Input: part model. Units: mm. Frame: model coordinates. A direction names the side the tool comes from. Coordinates: 2 decimals unless noted, no trailing zeros. Write each loop counter-clockwise with the first axis right and the second up, starting at its lowest first coordinate (ties: lowest second). Pieces come first, ordered by that corner, then holes. Notation, with made-up numbers: M 45.25,-1 L 86.25,-1 A10 ccw 86.25,3 Z; hole C 68.25,9 d5. An arc over 180 degrees is marked long. Use CSV: the item, a comma, the result in double quotes.
Autodesk Inventor part; units mm, degrees
ref_plane "YZ Plane" through (0, 0, 0) normal (1, 0, 0) x (0, 1, 0)
ref_plane "XZ Plane" through (0, 0, 0) normal (0, 1, 0) x (-1, 0, 0)
ref_plane "XY Plane" through (0, 0, 0) normal (0, 0, 1) x (1, 0, 0)
sketch "esq_rev" plane through (0, 0, 0) normal (0, 0, 1) x (1, 0, 0)
  line L0 (0, -38.1) -> (0, 50.1)
  line L1 (7.5, -9.5) -> (7.5, 9.5)
  line L2 (7.5, 9.5) -> (13, 9.5)
  line L3 (13, 9.5) -> (13, 22.5)
  line L4 (13, 22.5) -> (30, 22.5)
  line L5 (30, 22.5) -> (30, 37.5)
  line L6 (30, 37.5) -> (0, 37.5)
  line L7 (0, -25.5) -> (0, -0.0006)
  line L8 (-38.091, 0) -> (41.3485, 0)
  line L9 (-26.7425, 30) -> (-5.3911, 30)
  line L10 (-5.3911, 30) -> (28.4337, 30)
  line L11 (28.4337, 30) -> (7.0823, 30)
  line L12 (7.0823, 30) -> (-26.7425, 30)
  line L13 (-6.854, 30) -> (-23.5883, 30)
  line L14 (-23.5883, 30) -> (-14.3845, 30)
  line L15 (-4.5388, 30) -> (-6.854, 30)
  line L16 (-24.4454, 30) -> (5.2291, 30)
  line L17 (5.2291, 30) -> (2.6006, 30)
  line L18 (-13.9964, 30) -> (-24.4454, 30)
  line L19 (24.4454, 30) -> (-5.2291, 30)
  line L20 (-5.2291, 30) -> (-2.6006, 30)
  line L21 (13.9964, 30) -> (24.4454, 30)
  line L22 (4.5388, 30) -> (7.194, 30)
  line L23 (7.194, 30) -> (24.9396, 30)
  line L24 (24.9396, 30) -> (14.3845, 30)
  line L25 (-4.5388, 30) -> (-14.5, 30)
  line L26 (2.6006, 30) -> (-13.9964, 30)
  line L27 (13.9964, 30) -> (-2.6006, 30)
  line L28 (14.5, 30) -> (4.5388, 30)
  line L29 (-12.5, 30) -> (12.5, 30)
  line L30 (-12.5, -20) -> (12.5, -20)
  line L31 (7, -9.5) -> (7, -25.5)
  line L32 (7, -25.5) -> (0, -25.5)
  line L33 (7, -9.5) -> (7.5, -9.5)
  line L34 (0, -0.0006) -> (0, 37.5)
  point P0 (0, 0)
  dimension "d0" = 30
  dimension "d1" = 13
  dimension "d2" = 7.5
  dimension "d5" = 13
  dimension "d6" = 15
  dimension "d23" = 7
  dimension "d25" = 19
  dimension "d26" = 16
revolve "rev" add sketch "esq_rev" angle 360 about axis through (0, -25.5, 0) along (0, 1, 0)
sketch "esq_percage" plane through (0, 0, 0) normal (0, 1, 0) x (-1, 0, 0)
  line L0 (0, -7) -> (0, 7)
  line L1 (-7, 0) -> (7, 0)
  circle A0 centre (0, 0) radius 5
  dimension "d8" = 10
extrude "ext_percage" cut sketch "esq_percage" along normal through all both and the other way through all
sketch "Esq_trous" plane through (0, 0, 0) normal (0, 1, 0) x (-1, 0, 0)
  line L0 (0, -4.9) -> (0, 29.4)
  line L1 (-3.5, 0) -> (3.5, 0)
  circle A0 centre (0, 22) radius 2.5
  point P0 (0, 0)
  dimension "d11" = 5
  dimension "d12" = 22
extrude "ext_trous" cut sketch "Esq_trous" along normal through all
pattern_circular "Réseau circulaire1" count 6 over 360 about axis through (0, -10, 0) along (0, 1, 0) of "ext_trous"
thread "Filetage2"
properties part number "wheel_hub_spacer" material "Aluminium 6061"
1. Section A-A (z = 0). Return loops of the section in (x, y), then the cut area to 3 significant figures.
Resolved:
outline,"M -30,22.5 L -13,22.5 L -13,9.5 L -7.5,9.5 L -7.5,-9.5 L -7,-9.5 L -7,-25.5 L -5,-25.5 L -5,37.5 L -30,37.5 Z; M 5,-25.5 L 7,-25.5 L 7,-9.5 L 7.5,-9.5 L 7.5,9.5 L 13,9.5 L 13,22.5 L 30,22.5 L 30,37.5 L 5,37.5 Z"
area,"1,120 mm^2"
2. Section B-B (x = 0). Return loops of the section in (y, z), then the cut area to 3 significant figures.
Resolved:
outline,"M -25.5,-7 L -9.5,-7 L -9.5,-7.5 L 9.5,-7.5 L 9.5,-13 L 22.5,-13 L 22.5,-19.5 L 37.5,-19.5 L 37.5,-5 L -25.5,-5 Z; M -25.5,5 L 37.5,5 L 37.5,19.5 L 22.5,19.5 L 22.5,13 L 9.5,13 L 9.5,7.5 L -9.5,7.5 L -9.5,7 L -25.5,7 Z; M 22.5,-30 L 37.5,-30 L 37.5,-24.5 L 22.5,-24.5 Z; M 22.5,24.5 L 37.5,24.5 L 37.5,30 L 22.5,30 Z"
area,"967 mm^2"
3. Mould query, pull axis X, two halves, no side actions, for faces 1 (the flat face through (-2, -25.5, -5)), 2 (the cylindrical face through (-19.59, 29.9, 8.56)), 3 (the cylindrical face through (6.466, -17.612, -2.681)). Classes: pulls with the +X half, pulls with the -X half, needs draft (parallel to the pull), parting line crosses it, or undercut.
Resolved:
face 1,"needs draft"
face 2,"undercut"
face 3,"parting line crosses it"
4. Section D-D (y = 30). Return loops of the section in (x, z).
Resolved:
outline,"C 0,0 d60; hole C -19.05,-11 d5; hole C -19.05,11 d5; hole C 0,0 d10; hole C 0,-22 d5; hole C 0,22 d5; hole C 19.05,-11 d5; hole C 19.05,11 d5"
5. Access query for faces 4 (the cylindrical face through (1.08, 6.44, -4.88)), 5 (the flat face through (7, -9.5, -2)). Directions: +Z, -Z, +X, -X, +Y, -Y. A direction counts if a zero-diameter tool reaches every point of the face in a straight line with its end or side. Return the directions, or none.
Resolved:
face 4,"+Y, -Y"
face 5,"-Y"
6. Contact query for flat-ended pins moving along their axis: pin 1 Ø6.5 at (x, z) = (0, 22) entering from +Y; pin 2 Ø10 at (x, z) = (22, -21) entering from -Y; pin 3 Ø1.5 at (y, z) = (28, -3.5) entering from +X; pin 4 Ø2 at (x, y) = (-11, 17) entering from +Z. Output: stop coordinate, or through.
Resolved:
pin 1,"stops at y = 37.5"
pin 2,"stops at y = 22.5"
pin 3,"stops at x = 29.87"
pin 4,"stops at z = 8.31"
7. Section C-C (y = 2.5). Return loops of the section in (x, z), then the cut area to 3 significant figures.
Resolved:
outline,"C 0,0 d15; hole C 0,0 d10"
area,"98.2 mm^2"
8. Material intervals for line 1 (Z direction, x = 0, y = 6); line 2 (Y direction, x = -10, z = 4); line 3 (Y direction, x = -14.5, z = 17.5), sorted ascending. Write a range as [from, to].
Resolved:
line 1,"z = [-7.5, -5], [5, 7.5]"
line 2,"y = [9.5, 37.5]"
line 3,"y = [22.5, 37.5]"
